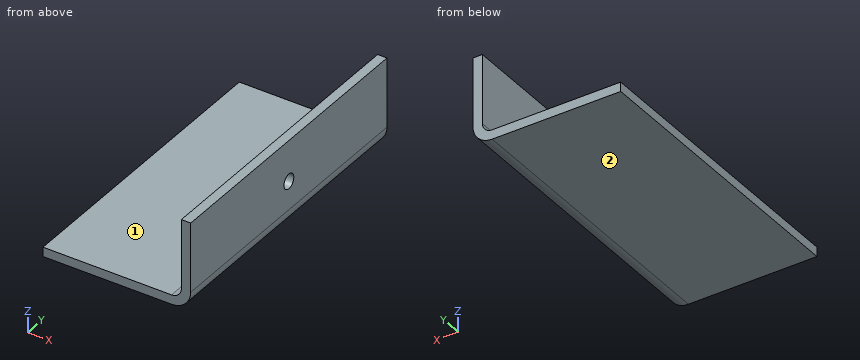
from build123d import *

# Parameters (mm, degrees)
SKETCH1_W                    = 50
SKETCH1_H                    = 100
BASE_FLANGE2_DEPTH           = 3.175
EDGE_FLANGE1_STRIP_W         = 19.304
EDGE_FLANGE1_STRIP_H         = 3.175
EDGE_FLANGE1_STRIP_CUT_DEPTH = 100
EDGE_FLANGE1_DEPTH           = 100
F_5_0MM_DOWEL_HOLE1_D        = 5


# Sheet-metal steps are written as plain solids
with BuildPart() as part:
    # Sketch1 → Base-Flange2 (new body)
    with BuildSketch(Plane.XY):
        Rectangle(SKETCH1_W, SKETCH1_H)
    extrude(amount=-BASE_FLANGE2_DEPTH)

    # Edge-Flange1 strip (across the edge) → Edge-Flange1 strip cut (cut)
    with BuildSketch(Plane(origin=(25, -50, 0), x_dir=(-1, 0, 0), z_dir=(0, 1, 0))):
        with Locations((-3.175, -1.5875)):
            Rectangle(EDGE_FLANGE1_STRIP_W, EDGE_FLANGE1_STRIP_H)
    extrude(amount=EDGE_FLANGE1_STRIP_CUT_DEPTH, mode=Mode.SUBTRACT)

    # Edge-Flange1 section (across the edge) → Edge-Flange1 (add)
    with BuildSketch(Plane(origin=(25, -50, 0), x_dir=(-1, 0, 0), z_dir=(0, 1, 0))):
        with BuildLine():
            Line((0, 3.302), (0, 26.825))
            Line((0, 26.825), (3.175, 26.825))
            Line((3.175, 26.825), (3.175, 3.302))
            ThreePointArc((3.175, 3.302), (4.142133409, 0.967133409), (6.477, 0))
            Line((6.477, 0), (6.477, -3.175))
            ThreePointArc((6.477, -3.175), (1.897069378, -1.277930622), (0, 3.302))
        make_face()
    extrude(amount=EDGE_FLANGE1_DEPTH)

    # Ø5.0mm Dowel Hole1 (through all)
    with Locations(Plane(origin=(25, 0, 0), x_dir=(0, 0, -1), z_dir=(1, 0, 0))):
        with Locations((-12.954, 0)):
            Hole(F_5_0MM_DOWEL_HOLE1_D / 2)


solid = part.part
Design review of the part built by this model. Coordinates are the model's own, in mm. Face numbers are marked on the shaded views. A direction names the side the tool comes from. Coordinates: 2 decimals unless noted, no trailing zeros. Order: outer loops, then holes, each group sorted by start corner. A loop starts at its lowest first (then second) coordinate and runs counter-clockwise, first axis right, second up. Notation, with made-up numbers: M 68,22.25 L 112,22.25 A21 ccw 112,52.25 Z; hole C 52.25,80.5 d9. An arc over 180 degrees is marked long. Use a Markdown table: item, result.
(1) Add section C-C (x = 2). Give the boundary of the cut face in (y, z) (3 decimals), then the cut area to 4 significant figures.
Worked answers:
| item | result |
|---|---|
| outline | M -50,-3.175 L 50,-3.175 L 50,0 L -50,0 Z |
| area | 317.5 mm2 |
(2) For P1, Ø7, axis at y = -6.5, z = 13, coming from the -X side (3 decimals); P2, Ø6, axis at x = 8, y = 15.5, coming from the +Z side; P3, Ø8, axis at x = 5, z = 2, coming from the -Y side; P4, Ø4.5, axis at y = 0, z = 12.954, coming from the +X side, all flat-tipped, find the tip position at first contact; note any pin that passes through.
Worked answers:
| item | result |
|---|---|
| P1 | stops at x = 21.825 |
| P2 | stops at z = 0 |
| P3 | stops at y = -50 |
| P4 | passes through |
(3) Wall thickness on probe 1 along X at (y, z) = (3, 7) (3 decimals); probe 2 along Z at (x, y) = (-11, -4) (3 decimals); probe 3 along X at (y, z) = (34, 1): over which ranges is each line inside the solid? List them lowest first.
Worked answers:
| item | result |
|---|---|
| probe 1 | x = 21.825 to 25 |
| probe 2 | z = -3.175 to 0 |
| probe 3 | x = 20.89 to 24.58 |
(4) For the marked faces 1 and 2, list the 3-axis set-ups (+Z, -Z, +X, -X, +Y, -Y) from which the entire face can be reached by the end or side of a thin tool; tool diameter is ignored.
Worked answers:
| item | result |
|---|---|
| face 1 | +Z, -X, +Y, -Y |
| face 2 | -Z, +X, -X, +Y, -Y |
(5) Add section A-A (y = 0). Give the boundary of the cut face in (x, z) (3 decimals).
Worked answers:
| item | result |
|---|---|
| outline | M -25,-3.175 L 18.523,-3.175 A6.477 ccw 25,3.302 L 25,10.454 L 21.825,10.454 L 21.825,3.302 A3.302 cw 18.523,0 L -25,0 Z; M 21.825,15.454 L 25,15.454 L 25,26.825 L 21.825,26.825 Z |
(6) Add section B-B (z = 23.75). Give the boundary of the cut face in (x, y) (3 decimals).
Worked answers:
| item | result |
|---|---|
| outline | M 21.825,-50 L 25,-50 L 25,50 L 21.825,50 Z |
